Source: CAD feature listing. Evaluate the final solid. Frame: model axes, mm. Round coordinates to 2 decimals unless told otherwise and drop trailing zeros. Write each loop counter-clockwise with the first axis right and the second up, starting at its lowest first coordinate (ties: lowest second). Pieces come first, ordered by that corner, then holes. Notation, with made-up numbers: M 2.25,-29 L 17.25,-29 A22 ccw 17.25,-11 Z; hole C 5,0.25 d11. An arc over 180 degrees is marked long. Use a Markdown table: item, result.
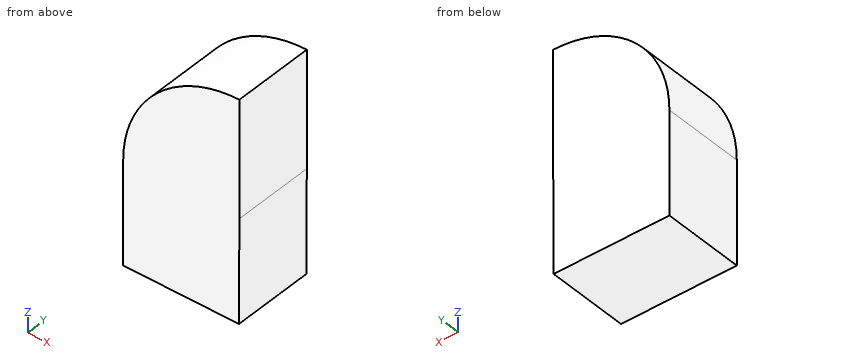
```python
from build123d import *

# Parameters (mm, degrees)
F1_DEPTH  = 25.4
F1_FACE_W = 72.2126737237
F1_FACE_H = 50.8
F2_ANGLE  = 90


with BuildPart() as f1:
    # F0 (on Front) → F1 (new body, symmetric)
    with BuildSketch(Plane.XZ):
        Polygon((0, 63.9712512493), (0, 0), (71.9514414668, 0), (72.2126737237, 63.9712512493), align=None)
    extrude(amount=F1_DEPTH, both=True)

    # F1_face (on face) → F2 (revolve)
    with BuildSketch(Plane(origin=(36.1063368618, 0, 63.9712512493), x_dir=(1, 0, 0), z_dir=(0, 0, 1))):
        Rectangle(F1_FACE_W, F1_FACE_H)
    revolve(axis=Axis((72.2126737237, 0, 63.9712512493), (0, 1, 0)), revolution_arc=F2_ANGLE)


solid = f1.part
```
Q1. First-contact query: pin 1 Ø4 at (x, y) = (48, 1.5) entering from +Z; pin 2 Ø3 at (x, y) = (53, 17) entering from +Z; pin 3 Ø2 at (x, y) = (25.5, -10.5) entering from -Z; pin 4 Ø8 at (x, y) = (17, 3.5) entering from +Z. Flat tips, straight axial feed; report the tip coordinate or a pass-through.
Results are:
| item | result |
|---|---|
| pin 1 | z = 132.68 |
| pin 2 | z = 133.98 |
| pin 3 | z = 0 |
| pin 4 | z = 114.88 |
Q2. Section A-A on y = 22. Return loops of the section in (x, z), plus the area to 3 significant figures.
Results are:
| item | result |
|---|---|
| outline | M 0,0 L 71.95,0 L 72.21,63.97 L 72.21,136.18 A72.21 ccw 0,63.97 Z |
| area | 8,710 mm^2 |
Q3. Section C-C on x = 48. Return loops of the section in (y, z).
Results are:
| item | result |
|---|---|
| outline | M -25.4,0 L 25.4,0 L 25.4,132 L -25.4,132 Z |
Q4. Section B-B on z = 78. Return loops of the section in (x, y), plus the area to 3 significant figures.
Results are:
| item | result |
|---|---|
| outline | M 1.38,-25.4 L 72.21,-25.4 L 72.21,25.4 L 1.38,25.4 Z |
| area | 3,600 mm^2 |
Q5. Line query: L1, parallel to X at y = -16.5, z = 65; L2, parallel to X at y = -9.5, z = 124; L3, parallel to Z at x = 31, y = -13.5. Output: solid intervals per line, ascending.
Results are:
| item | result |
|---|---|
| L1 | 0.01 to 72.21 |
| L2 | 32.07 to 72.21 |
| L3 | 0 to 123.27 |
